```python
from build123d import *

# Parameters (mm, degrees)
SALIENTE_EXTRUIR1_DEPTH = 20
CROQUIS2_R              = 2.25
CORTAR_EXTRUIR1_DEPTH   = 4
REDONDEO1_R             = 3


with BuildPart() as part:
    # Croquis1 → Saliente-Extruir1 (new body)
    with BuildSketch(Plane.XY):
        with BuildLine():
            Line((0, 0), (0, 22.5))
            ThreePointArc((0, 22.5), (-4, 26.5), (-8, 22.5))
            Line((-8, 22.5), (-8, 17.5))
            Line((-8, 17.5), (-12, 22.5))
            ThreePointArc((-12, 22.5), (-4, 30.5), (4, 22.5))
            Line((4, 22.5), (4, 4))
            Line((4, 4), (19, 4))
            Line((19, 4), (19, 0))
            Line((19, 0), (0, 0))
        make_face()
    extrude(amount=SALIENTE_EXTRUIR1_DEPTH)

    # Croquis2 → Cortar-Extruir1 (cut)
    with BuildSketch(Plane(origin=(0, 4, 0), x_dir=(1, 0, 0), z_dir=(0, 1, 0))):
        with Locations((11.5, -10)):
            Circle(CROQUIS2_R)
    extrude(amount=-CORTAR_EXTRUIR1_DEPTH, mode=Mode.SUBTRACT)

    # Redondeo1
    redondeo1_edges = [part.edges().sort_by_distance(p)[0] for p in [
        (-12, 22.5, 10),
        (4, 4, 10),
    ]]
    fillet(redondeo1_edges, radius=REDONDEO1_R)


solid = part.part
```
Check sheet for the modelled part. Datum: model origin and axes. Units: mm. A direction names the side the tool comes from. Coordinates: 2 decimals unless noted, no trailing zeros. Order: outer loops, then holes, each group sorted by start corner. A loop starts at its lowest first (then second) coordinate and runs counter-clockwise, first axis right, second up. Notation, with made-up numbers: (-9, 32) -> (21, 32) arc R9 cw to (21, 47) -> close; hole circle Ø5 at (12, -40). An arc over 180 degrees is marked (long way). Write item = value, one per line. Start each with the question number.
1) Cross-section at C-C (z = 17.25). Enter the section's corners in (x, y), then the cut area to 3 significant figures.
2) Go/stop test with flat-tipped pins: P1, Ø10, axis at y = 25, z = 4.5, coming from the +X side; P2, Ø12, axis at x = 4.5, y = 14.5, coming from the +Z side; P3, Ø6, axis at x = 10, z = 14.5, coming from the +Y side; P4, Ø8, axis at x = 5, z = 3.5, coming from the +Y side (3 decimals). Record where each tip stops, or that it passes through.
3) Access from +Z, -Z, +X, -X, +Y, -Y to the whole of each face (thin tool, end or side, straight path). Record for faces 1 (the flat face through (14, 4, 10)), 2 (the cylindrical face through (9.84, 2.03, 8.48)), 3 (the flat face through (-8, 20, 10)).
4) Cross-section at D-D (y = 11.5). Enter the section's corners in (x, z), then the cut area to 3 significant figures.
5) Cross-section at B-B (z = 10). Enter the section's corners in (x, y), then the cut area to 3 significant figures.
6) Material ranges on L1, parallel to Z at x = 11.5, y = 2.65; L2, parallel to X at y = 3, z = 10; L3, parallel to Y at x = 7.5, z = 7.75, recorded low to high.
7) Cross-section at A-A (x = 11.5). Enter the section's corners in (y, z).
Ans:
q1.outline = (-11.86, 24.01) arc R3 ccw to (-11.25, 21.57) -> (-8, 17.5) -> (-8, 22.5) arc R4 cw to (0, 22.5) -> (0, 0) -> (19, 0) -> (19, 4) -> (7, 4) arc R3 cw to (4, 7) -> (4, 22.5) arc R8 ccw to start
q1.area = 237 mm²
q2.P1 = 4
q2.P2 = 20
q2.P3 = 4
q2.P4 = 28.745
q3.face_1 = +Z, -Z, +X, +Y
q3.face_2 = +Y, -Y
q3.face_3 = +Z, -Z, -Y
q4.outline = (0, 0) -> (4, 0) -> (4, 20) -> (0, 20) -> close
q4.area = 80.0 mm²
q5.outline = (-11.86, 24.01) arc R3 ccw to (-11.25, 21.57) -> (-8, 17.5) -> (-8, 22.5) arc R4 cw to (0, 22.5) -> (0, 0) -> (9.25, 0) -> (9.25, 4) -> (7, 4) arc R3 cw to (4, 7) -> (4, 22.5) arc R8 ccw to start; (13.75, 0) -> (19, 0) -> (19, 4) -> (13.75, 4) -> close
q5.area = 219 mm²
q6.L1 = 0 to 7.75, 12.25 to 20
q6.L2 = 0 to 9.25, 13.75 to 19
q6.L3 = 0 to 4
q7.outline = (0, 0) -> (4, 0) -> (4, 7.75) -> (0, 7.75) -> close; (0, 12.25) -> (4, 12.25) -> (4, 20) -> (0, 20) -> close
